The listing builds one solid part. Answer for the finished solid, in the listing's coordinates (mm). A direction names the side the tool comes from. Round coordinates to 2 decimals unless told otherwise and drop trailing zeros. Write each loop counter-clockwise with the first axis right and the second up, starting at its lowest first coordinate (ties: lowest second). Pieces come first, ordered by that corner, then holes.
(1) A cutting plane is placed at A-A, the plane y = 0. Give the vertices of the cut face in (x, z), and give its area (3 significant figures).
(2) A cutting plane is placed at C-C, the plane z = -0.5. Give the vertices of the cut face in (x, y), and give its area (3 significant figures).
(3) The mould has two halves that part along Y. Classify faces 1 (the face through (-15.12, -11.59, 9.48)), 2 (the face through (0, -1, 9)), 3 (the face through (4, -12.4, 6.35)): +Y half, -Y half, draft (parallel to the pull), parting line (faces both ways), or undercut.
(4) Find the intervals of material crossed by probe 1 along Y at (x, z) = (0, -0.75); probe 2 along Y at (x, z) = (0, 10.5); probe 3 along Z at (x, y) = (-5, 4), in increasing order.
(5) For faces 4 (the face through (-0.1, 11.3, -3.112)), 5 (the face through (0, 0, 6.35)), 6 (the face through (0, 0, 3.888)), determine the directions among +Z, -Z, +X, -X, +Y, -Y from which every point of the face is accessible in a straight line to the end or side of a thin tool.
(6) A cutting plane is placed at D-D, the plane x = -4.5. Give the vertices of the cut face in (y, z), and give its area (3 significant figures).
(7) Each of these flat-tipped pins is pushed along its axis until it touches: pin 1 Ø3 at (x, z) = (4.5, 0.5) entering from -Y; pin 2 Ø4 at (x, z) = (-2, -0.5) entering from -Y; pin 3 Ø1.8 at (x, y) = (0, 0) entering from +Z; pin 4 Ø10 at (x, y) = (7.5, -6.5) entering from -Z. Where does it stop, or does it pass through?
from build123d import *

# Parameters (mm, degrees)
SKETCH2_R                = 12.7
BOSS_EXTRUDE1_DEPTH      = 6.35
BOSS_EXTRUDE1_DEPTH_BACK = 3.1115
SKETCH4_R                = 19.05
SKETCH4_R_2              = 1
BOSS_EXTRUDE2_DEPTH      = 6.35
SKETCH5_R                = 11
CUT_EXTRUDE1_DEPTH       = 7


with BuildPart() as part:
    # Sketch2 → Boss-Extrude1 (new body, two sides)
    with BuildSketch(Plane.XY) as boss_extrude1_sk:
        Circle(SKETCH2_R)
    extrude(amount=BOSS_EXTRUDE1_DEPTH)
    extrude(boss_extrude1_sk.sketch, amount=-BOSS_EXTRUDE1_DEPTH_BACK)

    # Sketch4 → Boss-Extrude2 (add)
    with BuildSketch(Plane.XY.offset(6.35)):
        Circle(SKETCH4_R)
        Circle(SKETCH4_R_2, mode=Mode.SUBTRACT)
    extrude(amount=BOSS_EXTRUDE2_DEPTH)

    # Sketch5 → Cut-Extrude1 (cut)
    with BuildSketch(Plane(origin=(0, 0, -3.1115), x_dir=(-1, 0, 0), z_dir=(0, 0, -1))):
        Circle(SKETCH5_R)
    extrude(amount=-CUT_EXTRUDE1_DEPTH, mode=Mode.SUBTRACT)


solid = part.part
Solutions:
1. outline: (-19.05, 6.35) - (-12.7, 6.35) - (-12.7, -3.11) - (-11, -3.11) - (-11, 3.89) - (11, 3.89) - (11, -3.11) - (12.7, -3.11) - (12.7, 6.35) - (19.05, 6.35) - (19.05, 12.7) - (1, 12.7) - (1, 6.35) - (-1, 6.35) - (-1, 12.7) - (-19.05, 12.7) - close
1. area: 316 mm2
2. outline: circle Ø25.4 at (0, 0); hole circle Ø22 at (0, 0)
2. area: 127 mm2
3. face 1: parting line
3. face 2: undercut
3. face 3: draft
4. probe 1: y = -12.7 to -11, 11 to 12.7
4. probe 2: y = -19.05 to -1, 1 to 19.05
4. probe 3: z = 3.89 to 12.7
5. face 4: -Z, +X, -X, +Y, -Y
5. face 5: +Z
5. face 6: -Z
6. outline: (-18.51, 6.35) - (-11.88, 6.35) - (-11.88, -3.11) - (-10.04, -3.11) - (-10.04, 3.89) - (10.04, 3.89) - (10.04, -3.11) - (11.88, -3.11) - (11.88, 6.35) - (18.51, 6.35) - (18.51, 12.7) - (-18.51, 12.7) - close
6. area: 319 mm2
7. pin 1: stops at y = -12.34
7. pin 2: stops at y = -12.7
7. pin 3: stops at z = 6.35
7. pin 4: stops at z = -3.11
